Input: part model. Units: mm. Frame: model coordinates. Give positions to 0.01 mm unless a question says otherwise; leave off trailing zeros. Order: outer loops, then holes, each group sorted by start corner. A loop starts at its lowest first (then second) coordinate and runs counter-clockwise, first axis right, second up. Notation, with made-up numbers: (-23.75, 83) -> (-14.75, 83) arc R25 cw to (-14.75, 95) -> close; hole circle Ø6 at (-5.75, 21.5). An arc over 180 degrees is marked (long way). Use a Markdown table: item, result. Add a question column.
from build123d import *

# Parameters (mm, degrees)
SKETCH1_R           = 1
BOSS_EXTRUDE1_DEPTH = 70
SKETCH3_W           = 4.158474465
SKETCH3_H           = 4.275067207
CUT_EXTRUDE1_DEPTH  = 1
SKETCH4_R           = 0.8
CUT_EXTRUDE2_DEPTH  = 4


with BuildPart() as part:
    # Sketch1 → Boss-Extrude1 (new body)
    with BuildSketch(Plane.XY):
        with Locations((-6.504393421, -0.589738754)):
            Circle(SKETCH1_R)
    extrude(amount=BOSS_EXTRUDE1_DEPTH)

    # Sketch2 → Revolve1 (revolve)
    with BuildSketch(Plane(origin=(0, 0, -1), x_dir=(-1, 0, 0), z_dir=(0, 0, -1))):
        with BuildLine():
            Line((6.504393421, 1.410261246), (6.504393421, -2.589738754))
            ThreePointArc((6.504393421, -2.589738754), (4.504393421, -0.589738754), (6.504393421, 1.410261246))
        make_face()
    revolve(axis=Axis((-6.504393421, 2.047627036, -1), (0, -1, 0)))

    # Sketch3 → Cut-Extrude1 (cut)
    with BuildSketch(Plane(origin=(0, 0, 0), x_dir=(1, 0, 0), z_dir=(0, 1, 0))):
        with Locations((-6.409968211, -68.247716877)):
            Rectangle(SKETCH3_W, SKETCH3_H)
    extrude(amount=CUT_EXTRUDE1_DEPTH, mode=Mode.SUBTRACT)

    # Sketch4 → Cut-Extrude2 (cut)
    with BuildSketch(Plane(origin=(0, 0, 0), x_dir=(1, 0, 0), z_dir=(0, 1, 0))):
        with Locations(Location((-6.504393421, -68, 0), (0, 0, 270))):
            Circle(SKETCH4_R)
    extrude(amount=-CUT_EXTRUDE2_DEPTH, mode=Mode.SUBTRACT)


solid = part.part
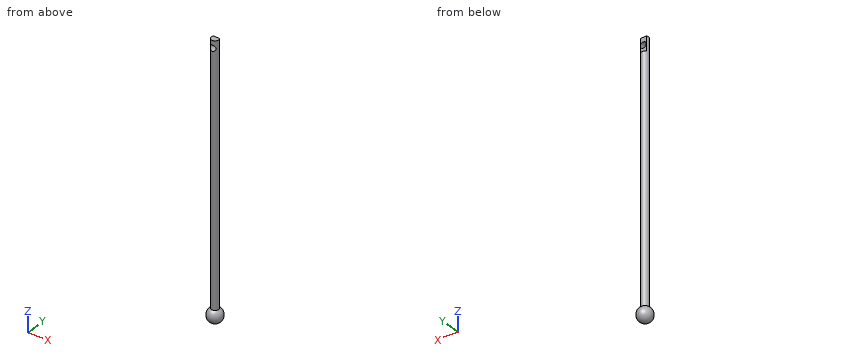
Q1. First-contact query: pin 1 (0.5 mm diameter, centred on x = -6.5, z = 67.5, fed in from +Y); pin 2 (2 mm diameter, centred on y = 1, z = 17, fed in from +X); pin 3 (1.5 mm diameter, centred on y = 0.5, z = 50.5, fed in from +X); pin 4 (1.8 mm diameter, centred on x = -6.5, z = 68, fed in from -Y). Flat tips, straight axial feed; report the tip coordinate or a pass-through.
Q2. Ray query, line 1 (X direction, y = -0.6, z = 68); line 2 (Y direction, x = -6.35, z = 42.5); line 3 (Y direction, x = -6.1, z = 44). Return the intervals inside material, ascending.
Q3. Section query B-B (z = 14). Return loops of the section in (x, y), plus the area to 3 significant figures.
Solution:
| question | item | result |
|---|---|---|
| 1 | pin 1 | passes through |
| 1 | pin 2 | stops at x = -5.7 |
| 1 | pin 3 | stops at x = -5.56 |
| 1 | pin 4 | stops at y = -1.59 |
| 2 | line 1 | x = -7.5 to -7.3, -5.7 to -5.5 |
| 2 | line 2 | y = -1.58 to 0.4 |
| 2 | line 3 | y = -1.5 to 0.32 |
| 3 | outline | circle Ø2 at (-6.5, -0.59) |
| 3 | area | 3.14 mm² |
